Autodesk Inventor part; units mm, degrees
ref_plane "YZ Plane" through (0, 0, 0) normal (1, 0, 0) x (0, 1, 0)
ref_plane "XZ Plane" through (0, 0, 0) normal (0, 1, 0) x (-1, 0, 0)
ref_plane "XY Plane" through (0, 0, 0) normal (0, 0, 1) x (1, 0, 0)
sketch "Sketch1" plane through (0, 0, 0) normal (0, 0, 1) x (1, 0, 0)
  line L0 (0, 0) -> (6, 0)
  line L1 (6, 0) -> (6, -20)
  line L2 (0, 0) -> (-6, 0)
  line L3 (-6, 0) -> (-6, 20)
  circle A0 centre (-6, 20) radius 2
  circle A1 centre (-6, 20) radius 1.25
  line L4 (-6, 0) -> (-6, 10)
  circle A2 centre (-6, 10) radius 1.25
  circle A3 centre (6, 0) radius 2
  circle A4 centre (-6, 0) radius 2
  line L5 (-8, 20) -> (-8, 0)
  line L6 (-4, 20) -> (-4, 2.5)
  line L7 (-6, -2) -> (3.5, -2)
  line L8 (-3.5, 2) -> (6, 2)
  circle A5 centre (6, -20) radius 2
  line L9 (4, -20) -> (4, -2.5)
  line L10 (8, 0) -> (8, -20)
  arc A6 (-4, 2.5) -> (-3.5, 2) centre (-3.5, 2.5) ccw
  arc A7 (4, -2.5) -> (3.5, -2) centre (3.5, -2.5) ccw
  line L11 (-8, 20) -> (-4, 20)
  line L12 (-4, 20) -> (-4, 16)
  line L13 (-4, 16) -> (-8, 16)
  line L14 (-8, 16) -> (-8, 20)
  arc A8 (-4, 16) -> (-8, 16) centre (-6, 13.7639) ccw
  line L15 (-4, 10) -> (-8, 10)
  line L16 (-8, 10) -> (-8, 14)
  line L17 (-8, 14) -> (-4, 14)
  line L18 (-4, 14) -> (-4, 10)
  line L19 (-4, 10) -> (-8, 10)
  line L20 (-8, 10) -> (-8, 6)
  line L21 (-8, 6) -> (-4, 6)
  line L22 (-4, 6) -> (-4, 10)
  arc A9 (-8, 14) -> (-4, 14) centre (-6, 16.2361) ccw
  arc A10 (-4, 6) -> (-8, 6) centre (-6, 3.7639) ccw
  line L23 (6, 0) -> (6, -7)
  circle A11 centre (6, -7) radius 1.25
  line L24 (6, -20) -> (6, -13)
  circle A12 centre (6, -13) radius 1.25
  line L25 (4, -6.5) -> (4, -3.5)
  line L26 (8, -3.5) -> (8, -6.5)
  line L27 (4, -13.5) -> (4, -16.5)
  line L28 (8, -16.5) -> (8, -13.5)
  line L29 (8, -7) -> (4, -7)
  line L30 (4, -7) -> (4, -4)
  line L31 (4, -4) -> (8, -4)
  line L32 (8, -4) -> (8, -7)
  line L33 (8, -13) -> (4, -13)
  line L34 (4, -13) -> (4, -16)
  line L35 (4, -16) -> (8, -16)
  line L36 (8, -16) -> (8, -13)
  point P0 (-4, 0)
  point P1 (6, -2)
  point P2 (-6, 2)
  point P3 (6, 2)
  point P4 (4, 0)
  point P5 (-4, 6)
  point P6 (-4, 14)
  point P7 (-8, 16)
  point P8 (4, -4)
  point P9 (4, -16)
  point P10 (8, -16)
  dimension "d44" = 6
  dimension "d45" = 20
  dimension "d46" = 6
  dimension "d47" = 20
  dimension "d48" = 4
  dimension "d49" = 2.5
  dimension "d50" = 10
  dimension "d51" = 2.5
  dimension "d52" = 4
  dimension "d53" = 4
  dimension "d54" = 4
  dimension "d55" = 0.5
  dimension "d56" = 0.5
  dimension "d57" = 4
  dimension "d58" = 20
  dimension "d59" = 3
  dimension "d60" = 4
  dimension "d61" = 10
  dimension "d62" = 4
  dimension "d63" = 3
  dimension "d64" = 3
  dimension "d66" = 2.5
  dimension "d68" = 2.5
  dimension "d75" = 7
  dimension "d77" = 7
  dimension "d78" = 3
  dimension "d79" = 3
extrude "Extrusion8" add sketch "Sketch1" along normal mid plane 4 contours L2 A4 L3 L21 L6 A6 L8 A3 L0 | L0 A3 L1 L31 L9 A7 L7 A4 L2 | A3 L1 L0 | L0 L1 A3 | A4 L3 L2 | L2 L3 A4 | A3 L10 L31 L1 | A4 L5 L21 L3 | L31 L10 L29 A11 L1 | L1 A11 L29 L9 L31 | L21 A10 L3 | L3 A10 L21 | L5 L15 A2 L3 A10 | L3 A2 L15 L6 A10 | L29 L10 L33 A12 L1 A11 | A11 L1 A12 L33 L9 L29 | L5 A9 L3 A2 L15 | L15 A2 L3 A9 L6 | L5 L13 L3 L17 | L17 L3 A9 | L17 L3 L13 L6 | A9 L3 L17 | L10 L35 L1 A12 L33 | L33 A12 L1 L35 L9 | A8 L3 L13 | L5 A0 L3 A8 | A8 L3 A0 L6 | L13 L3 A8 | L11 A1 L3 A0 | A0 L11 A1 | A0 L3 A1 L11 | L10 A5 L1 L35 | L35 L1 A5 L9 | A5
extrude "Extrusion9" cut sketch "Sketch1" along normal mid plane 2 contours L31 L10 L29 A11 L1 | L1 A11 L29 L9 L31 | L5 L15 A2 L3 A10 | L3 A2 L15 L6 A10 | L29 L10 L33 A12 L1 A11 | A11 L1 A12 L33 L9 L29 | L5 A9 L3 A2 L15 | L15 A2 L3 A9 L6 | L10 L35 L1 A12 L33 | L33 A12 L1 L35 L9 | L5 A0 L3 A8 | A8 L3 A0 L6 | L11 A1 L3 A0 | A0 L11 A1 | A0 L3 A1 L11
properties part number "link7" material "Aluminum 6061"
Source: CAD feature listing. Evaluate the final solid. Frame: model axes, mm. A direction names the side the tool comes from. Coordinates: 2 decimals unless noted, no trailing zeros. Loops run counter-clockwise (first coordinate to the right, second up) from the corner with the lowest first, then second, coordinate; pieces in that order, holes last. Notation, with made-up numbers: (86.25, 56.25) - (99.25, 56.25) arc R8 ccw to (99.25, 61.25) - close; hole circle Ø4 at (60.25, 46). An arc over 180 degrees is marked (long way). One line per item, written item: value. Start each with the question number.
1. Mould query, pull axis Y, two halves, no side actions, for faces 3 (the flat face through (1, 2, 0)), 4 (the cylindrical face through (5.01, -6.24, -1.51)), 5 (the flat face through (-1, -2, 0)), 6 (the flat face through (0, 0, -2)). Classes: pulls with the +Y half, pulls with the -Y half, needs draft (parallel to the pull), parting line crosses it, or undercut.
2. Ray query, L1, parallel to Y at x = -6, z = -1.4; L2, parallel to Y at x = 6, z = -1.7; L3, parallel to X at y = 20, z = 1.3. Return the intervals inside material, ascending.
3. Section A-A (z = -0.6). Return the cut outline in (x, y).
4. Contact query for flat-ended pins moving along their axis: P1, Ø6, axis at x = -2.5, y = 3, coming from the +Z side; P2, Ø1.6, axis at x = 7, z = 0, coming from the -Y side; P3, Ø2, axis at x = -6, y = 20, coming from the +Z side; P4, Ø1, axis at x = 5.5, z = 0, coming from the +Y side. Output: stop coordinate, or through.
5. Section C-C (z = 1.4). Return the cut outline in (x, y), and give its area (3 significant figures).
6. Section B-B (y = -13). Return the cut outline in (x, z).
7. Set-up query: faces 1 (the cylindrical face through (-6.921, 9.155, 1.493)), 2 (the flat face through (6, -4, 0)). Return all of +Z, -Z, +X, -X, +Y, -Y with unobstructed straight access to the full face (end or side cutting, diameter ignored); none if empty.
8. Section D-D (y = 15). Return the cut outline in (x, z).
Verdict:
1. face 3: pulls with the +Y half
1. face 4: undercut
1. face 5: pulls with the -Y half
1. face 6: needs draft
2. L1: y = -2 to 8.75, 11.25 to 18.75, 21.25 to 22
2. L2: y = -22 to -14.25, -11.75 to -8.25, -5.75 to 2
2. L3: x = -8 to -7.25, -4.75 to -4
3. outline: (-8, 0) arc R2 ccw to (-6, -2) - (3.5, -2) arc R0.5 cw to (4, -2.5) - (4, -4) - (8, -4) - (8, 0) arc R2 ccw to (6, 2) - (-3.5, 2) arc R0.5 cw to (-4, 2.5) - (-4, 6) arc R3 ccw to (-8, 6) - close; (-8, 14) arc R3 ccw to (-4, 14) - (-4, 16) arc R3 ccw to (-8, 16) - close; (4, -20) arc R2 ccw to (8, -20) - (8, -16) - (4, -16) - close
4. P1: stops at z = 2
4. P2: stops at y = -21.99
4. P3: passes through
4. P4: stops at y = 2
5. outline: (-8, 0) arc R2 ccw to (-6, -2) - (3.5, -2) arc R0.5 cw to (4, -2.5) - (4, -20) arc R2 ccw to (8, -20) - (8, 0) arc R2 ccw to (6, 2) - (-3.5, 2) arc R0.5 cw to (-4, 2.5) - (-4, 20) arc R2 ccw to (-8, 20) - close; hole circle Ø2.5 at (-6, 10); hole circle Ø2.5 at (-6, 20); hole circle Ø2.5 at (6, -13); hole circle Ø2.5 at (6, -7)
5. area: 199 mm2
6. outline: (4, -2) - (4.75, -2) - (4.75, -1) - (4, -1) - close; (4, 1) - (4.75, 1) - (4.75, 2) - (4, 2) - close; (7.25, -2) - (8, -2) - (8, -1) - (7.25, -1) - close; (7.25, 1) - (8, 1) - (8, 2) - (7.25, 2) - close
7. face 1: +Z, -Z
7. face 2: +X, -X
8. outline: (-8, -2) - (-4, -2) - (-4, 2) - (-8, 2) - close
